```python
from build123d import *

# Parameters (mm, degrees)
MODEL_W             = 6
MODEL_H             = 6
BOSS_EXTRUDE1_DEPTH = 6


with BuildPart() as part:
    # Model → Boss-Extrude1 (new body)
    with BuildSketch(Plane.XY):
        with BuildLine():
            Line((3925.531656445, 1073.487893097), (3916.031656445, 1073.487893097))
            Line((3916.031656445, 1073.487893097), (3916.0316001, 1076.513895594))
            Line((3916.0316001, 1076.513895594), (3910.0316001, 1076.513895594))
            Line((3910.0316001, 1076.513895594), (3910.0316001, 1073.513895594))
            Line((3910.0316001, 1073.513895594), (3898.031656445, 1073.487893097))
            Line((3898.031656445, 1073.487893097), (3898.031656445, 1076.487893097))
            Line((3898.031656445, 1076.487893097), (3892.031656445, 1076.487893097))
            Line((3892.031656445, 1076.487893097), (3892.031656445, 1073.487893097))
            Line((3892.031656445, 1073.487893097), (3882.531656445, 1073.487893097))
            ThreePointArc((3882.531656445, 1073.487893097), (3904.031656445, 1094.987893097), (3925.531656445, 1073.487893097))
        make_face()
        with Locations((3904.0316001, 1086.513895594)):
            Rectangle(MODEL_W, MODEL_H, mode=Mode.SUBTRACT)
    extrude(amount=BOSS_EXTRUDE1_DEPTH)


solid = part.part
```
The model under review builds one solid part; all positions refer to its coordinate system, in mm. A direction names the side the tool comes from. Give positions to 0.01 mm unless a question says otherwise; leave off trailing zeros. Write each loop counter-clockwise with the first axis right and the second up, starting at its lowest first coordinate (ties: lowest second). Pieces come first, ordered by that corner, then holes. Notation, with made-up numbers: (38.5, 33) - (91.5, 33) arc R33 ccw to (91.5, 72) - close; hole circle Ø2 at (4, 10). An arc over 180 degrees is marked (long way). Answer in a Markdown table with one row per item. Add a question column.
1. Wall thickness on line 1 along X through (y, z) = (1074.5, 0.65); line 2 along X through (y, z) = (1085, 0.85); line 3 along X through (y, z) = (1085.5, 0.3): over which ranges is each line inside the solid? List them lowest first. Write a range as [from, to].
2. We need section B-B on z = 2.45. Write out the cut boundary in (x, y), then the cut area to 3 significant figures.
3. Insertion check: P1, Ø1.5, axis at y = 1074.5, z = 2.5, coming from the -X side; P2, Ø2, axis at x = 3906, z = 3.5, coming from the -Y side; P3, Ø0.9, axis at y = 1074.5, z = 4, coming from the +X side; P4, Ø4, axis at x = 3892.5, y = 1083.5, coming from the -Z side. Each pin has a flat end and moves straight along its axis. Give the tip position at first contact, or say it passes through.
4. We need section D-D on y = 1092.5. Write out the cut boundary in (x, z).
5. Tool access review of faces 1 (the flat face through (3895, 1076.488, 3)), 2 (the flat face through (3904, 1082, 6)), 3 (the flat face through (3904, 1083.514, 3)): name each direction out of +Z, -Z, +X, -X, +Y, -Y from which nothing blocks a thin tool from reaching the whole face with its end or side.
6. Draft analysis for pull direction X (two halves, no side actions). For faces 4 (the flat face through (3921, 1073.488, 3)), 5 (the flat face through (3901.032, 1086, 3)), 6 (the cylindrical face through (3903.559, 1094.983, 2.958)), state which applies: +X half, -X half, draft (parallel to the pull), parting line (faces both ways), or undercut.
7. We need section C-C on x = 3896.5. Write out the cut boundary in (y, z), then the cut area to 3 significant figures.
8. We need section A-A on y = 1075. Write out the cut boundary in (x, z), then the cut area to 3 significant figures.
Ans:
| question | item | result |
|---|---|---|
| 1 | line 1 | x = [3882.56, 3892.03], [3898.03, 3910.03], [3916.03, 3925.51] |
| 1 | line 2 | x = [3885.87, 3901.03], [3907.03, 3922.19] |
| 1 | line 3 | x = [3886.2, 3901.03], [3907.03, 3921.86] |
| 2 | outline | (3882.53, 1073.49) - (3892.03, 1073.49) - (3892.03, 1076.49) - (3898.03, 1076.49) - (3898.03, 1073.49) - (3910.03, 1073.51) - (3910.03, 1076.51) - (3916.03, 1076.51) - (3916.03, 1073.49) - (3925.53, 1073.49) arc R21.5 ccw to start; hole (3901.03, 1083.51) - (3907.03, 1083.51) - (3907.03, 1089.51) - (3901.03, 1089.51) - close |
| 2 | area | 654 mm^2 |
| 3 | P1 | stops at x = 3882.53 |
| 3 | P2 | stops at y = 1073.5 |
| 3 | P3 | stops at x = 3925.52 |
| 3 | P4 | stops at z = 0 |
| 4 | outline | (3893.99, 0) - (3914.07, 0) - (3914.07, 6) - (3893.99, 6) - close |
| 5 | face 1 | +Z, -Z, -Y |
| 5 | face 2 | +Z, +X, -X, +Y, -Y |
| 5 | face 3 | +Z, -Z |
| 6 | face 4 | draft |
| 6 | face 5 | undercut |
| 6 | face 6 | parting line |
| 7 | outline | (1076.49, 0) - (1093.63, 0) - (1093.63, 6) - (1076.49, 6) - close |
| 7 | area | 103 mm^2 |
| 8 | outline | (3882.58, 0) - (3892.03, 0) - (3892.03, 6) - (3882.58, 6) - close; (3898.03, 0) - (3910.03, 0) - (3910.03, 6) - (3898.03, 6) - close; (3916.03, 0) - (3925.48, 0) - (3925.48, 6) - (3916.03, 6) - close |
| 8 | area | 185 mm^2 |
